Read the model definition and answer for the solid it produces. Units are mm, in the model's axes. Face numbers are marked on the shaded views. A direction names the side the tool comes from. Give positions to 0.01 mm unless a question says otherwise; leave off trailing zeros. Write each loop counter-clockwise with the first axis right and the second up, starting at its lowest first coordinate (ties: lowest second). Pieces come first, ordered by that corner, then holes. Notation, with made-up numbers: (0, 57.5) -> (18, 57.5) arc R21 ccw to (18, 73.5) -> close; hole circle Ø3 at (-8, 21.25). An arc over 180 degrees is marked (long way). Use a Markdown table: item, result.
from build123d import *

# Parameters (mm, degrees)
ESQUISSE1_W                  = 9
ESQUISSE1_H                  = 63
BOSS_EXTRU_1_DEPTH           = 10
ESQUISSE2_W                  = 5
ESQUISSE2_H                  = 63
BOSS_EXTRU_2_DEPTH           = 63
CONG_3_R                     = 1
CONG_4_R                     = 1
CONG_5_R                     = 1
CONG_6_R                     = 1
ESQUISSE3_R                  = 2.5
ENL_V_MAT_EXTRU_1_DEPTH      = 77.075062882
ENL_V_MAT_EXTRU_3_DEPTH      = 77.075062882
ENL_V_MAT_EXTRU_3_DEPTH_BACK = 77.075062882
ESQUISSE9_R                  = 2.5
ENL_V_MAT_EXTRU_4_DEPTH      = 23
ESQUISSE12_W                 = 9
ESQUISSE12_H                 = 63
BOSS_EXTRU_4_DEPTH           = 5
ESQUISSE13_R                 = 1.8
ENL_V_MAT_EXTRU_6_DEPTH      = 4
ENL_V_START                  = -4
ESQUISSE14_R                 = 1.8
ENL_V_MAT_EXTRU_7_DEPTH      = 4


with BuildPart() as part:
    # Esquisse1 → Boss.-Extru.1 (new body)
    with BuildSketch(Plane.XY):
        with Locations((-9.542944785, -10.564417178)):
            Rectangle(ESQUISSE1_W, ESQUISSE1_H)
    extrude(amount=BOSS_EXTRU_1_DEPTH)

    # Esquisse2 → Boss.-Extru.2 (add)
    with BuildSketch(Plane(origin=(0, 0, 0), x_dir=(-1, 0, 0), z_dir=(0, 0, -1))):
        with Locations((9.542944785, -10.564417178)):
            Rectangle(ESQUISSE2_W, ESQUISSE2_H)
    extrude(amount=BOSS_EXTRU_2_DEPTH)

    # Congé3
    cong_3_edges = [part.edges().sort_by_distance(p)[0] for p in [
        (-7.042944785, -10.564417178, 0),
    ]]
    fillet(cong_3_edges, radius=CONG_3_R)

    # Congé4
    cong_4_edges = [part.edges().sort_by_distance(p)[0] for p in [
        (-12.042944785, -10.564417178, 0),
    ]]
    fillet(cong_4_edges, radius=CONG_4_R)

    # Congé5
    cong_5_edges = [part.edges().sort_by_distance(p)[0] for p in [
        (-5.042944785, -10.564417178, 0),
    ]]
    fillet(cong_5_edges, radius=CONG_5_R - 0.0001)  # a hair under: the kernel refuses the full size

    # Congé6
    cong_6_edges = [part.edges().sort_by_distance(p)[0] for p in [
        (-14.042944785, -10.564417178, 0),
    ]]
    fillet(cong_6_edges, radius=CONG_6_R - 0.0001)  # a hair under: the kernel refuses the full size

    # Esquisse3 → Enlèv. mat.-Extru.1 (cut, through all)
    with BuildSketch(Plane.ZY.offset(12.042944785)):
        with Locations(Location((-43, -10.564417178, 0), (0, 0, 270))):
            Circle(ESQUISSE3_R)
    extrude(amount=-ENL_V_MAT_EXTRU_1_DEPTH, mode=Mode.SUBTRACT)

    # Esquisse7 → Enlèv. mat.-Extru.3 (cut, two sides: drawn at the far end of the back side and taken through both)
    with BuildSketch(Plane(origin=(-7.042944785, 0, 0), x_dir=(0, 0, -1), z_dir=(1, 0, 0)).offset(-ENL_V_MAT_EXTRU_3_DEPTH_BACK)):
        Polygon((51.248405369, 207.781395644), (51.248405369, 20.935582822), (51.248405369, -42.839359106), (51.248405369, -229.685171928), (424.940031013, -229.685171928), (424.940031013, 207.781395644), align=None)
    extrude(amount=ENL_V_MAT_EXTRU_3_DEPTH + ENL_V_MAT_EXTRU_3_DEPTH_BACK, mode=Mode.SUBTRACT)


with BuildPart() as body_2:
    # Fractionner1: the piece on the far side of the plane
    add(part.part)
    split(bisect_by=Plane.XY.offset(-31.402624734), keep=Keep.BOTTOM)


with BuildPart() as part_1:
    add(part.part)

    # Fractionner1
    split(bisect_by=Plane.XY.offset(-31.402624734), keep=Keep.TOP)

    # Esquisse9 → Enlèv. mat.-Extru.4 (cut)
    with BuildSketch(Plane(origin=(-7.042944785, 0, 0), x_dir=(0, 0, -1), z_dir=(1, 0, 0))):
        with Locations(Location((22.835321424, -10.036411033, 0), (0, 0, 90))):
            Circle(ESQUISSE9_R)
    extrude(amount=-ENL_V_MAT_EXTRU_4_DEPTH, mode=Mode.SUBTRACT)

    # Esquisse12 → Boss.-Extru.4 (add)
    with BuildSketch(Plane.XY.offset(10)):
        with Locations((-9.542944785, -10.564417178)):
            Rectangle(ESQUISSE12_W, ESQUISSE12_H)
    extrude(amount=BOSS_EXTRU_4_DEPTH)

    # Esquisse13 → Enlèv. mat.-Extru.6 (cut)
    with BuildSketch(Plane(origin=(0, 20.935582822, 0), x_dir=(1, 0, 0), z_dir=(0, 1, 0))):
        with Locations(Location((-9.5, -8, 0), (0, 0, 180))):
            Circle(ESQUISSE13_R)
    extrude(amount=-ENL_V_MAT_EXTRU_6_DEPTH, mode=Mode.SUBTRACT)

    # Esquisse14 → Enlèv. mat.-Extru.7 (cut)
    with BuildSketch(Plane(origin=(0, -42.064417178, 0), x_dir=(-1, 0, 0), z_dir=(0, -1, 0)).offset(ENL_V_START)):
        with Locations((9.5, -8)):
            Circle(ESQUISSE14_R)
    extrude(amount=ENL_V_MAT_EXTRU_7_DEPTH, mode=Mode.SUBTRACT)


solid = part_1.part
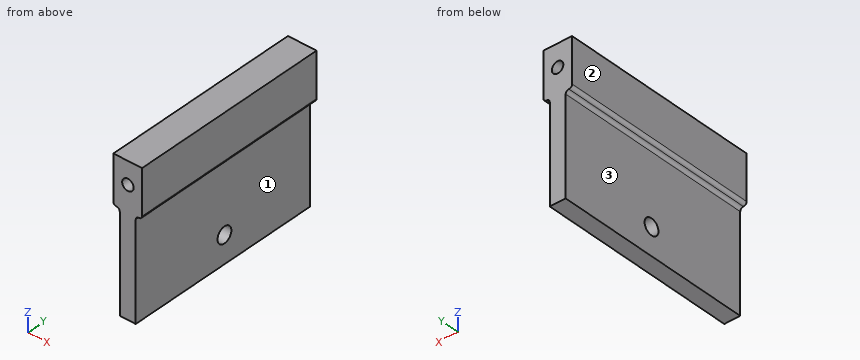
Item 1: Each of these flat-tipped pins is pushed along its axis until it touches: P1, Ø24.5, axis at y = -17.5, z = -20.5, coming from the +X side; P2, Ø2, axis at x = -9.5, z = 8, coming from the +Y side; P3, Ø3, axis at y = -22, z = -1, coming from the +X side; P4, Ø24.5, axis at y = -21.5, z = -10, coming from the -X side. Where does it stop, or does it pass through?
Return value:
| item | result |
|---|---|
| P1 | x = -7.04 |
| P2 | y = 16.94 |
| P3 | x = -5.18 |
| P4 | x = -14.04 |
Item 2: Straight lines are drawn through the part: line 1 along Z through (x, y) = (-9.5, 19.1); line 2 along X through (y, z) = (-9.5, -29); line 3 along X through (y, z) = (-39, 8). For each, find the intervals that lie inside material, in ascending order. Write a range as [from, to].
Return value:
| item | result |
|---|---|
| line 1 | [-31.4, 6.2], [9.8, 15] |
| line 2 | [-12.04, -7.04] |
| line 3 | [-14.04, -11.3], [-7.7, -5.04] |
Item 3: A cutting plane is placed at B-B (z = 8). Give the vertices of the cut face in (x, y), then the cut area to 3 significant figures.
Return value:
| item | result |
|---|---|
| outline | (-14.04, -42.06) -> (-11.3, -42.06) -> (-11.3, -38.06) -> (-7.7, -38.06) -> (-7.7, -42.06) -> (-5.04, -42.06) -> (-5.04, 20.94) -> (-7.7, 20.94) -> (-7.7, 16.94) -> (-11.3, 16.94) -> (-11.3, 20.94) -> (-14.04, 20.94) -> close |
| area | 538 mm^2 |
Item 4: A tool of negligible diameter and unlimited length cuts with its end or side. For the marked faces 1, 2 and 3, from which of +Z, -Z, +X, -X, +Y, -Y can it reach the whole face along a straight path? Write none if from no direction.
Return value:
| item | result |
|---|---|
| face 1 | -Z, +X, +Y, -Y |
| face 2 | +Z, -Z, -X, +Y, -Y |
| face 3 | -Z, -X, +Y, -Y |
Item 5: A cutting plane is placed at C-C (x = -9.5). Give the vertices of the cut face in (y, z).
Return value:
| item | result |
|---|---|
| outline | (-42.06, -31.4) -> (20.94, -31.4) -> (20.94, 6.2) -> (16.94, 6.2) -> (16.94, 9.8) -> (20.94, 9.8) -> (20.94, 15) -> (-42.06, 15) -> (-42.06, 9.8) -> (-38.06, 9.8) -> (-38.06, 6.2) -> (-42.06, 6.2) -> close; hole circle Ø5 at (-10.04, -22.84) |
